The listing builds one solid part. Answer for the finished solid, in the listing's coordinates (mm). A direction names the side the tool comes from. Give positions to 0.01 mm unless a question says otherwise; leave off trailing zeros. Order: outer loops, then holes, each group sorted by start corner. A loop starts at its lowest first (then second) coordinate and runs counter-clockwise, first axis right, second up. Notation, with made-up numbers: (-33.5, -19) - (-14.5, -19) arc R26 cw to (-14.5, 3) - close; hole circle Ø7 at (79.5, 59). An arc over 180 degrees is marked (long way). Answer as CSV lines item,"result". Start each with the question number.
1. Flat-ended cylindrical pins translate along their axes: pin 1 (2.5 mm diameter, centred on y = 29.5, z = -2, fed in from +X); pin 2 (2 mm diameter, centred on y = 24, z = -3.5, fed in from +X); pin 3 (4 mm diameter, centred on x = -52, y = 2, fed in from +Z); pin 4 (7.5 mm diameter, centred on x = 64.79, y = 11.18, fed in from +Z). Find the tip coordinate at first contact, or state that the pin passes through.
2. Section A-A on x = -2.5 is taken. Give the vertices of the cut face in (y, z), and give its area (3 significant figures).
3. Determine the mould class of faces 6 (the flat face through (-11, 26.183, 17)), 7 (the cylindrical face through (63.872, 7.034, 1.479)), 8 (the cylindrical face through (79.79, 11.51, 1.48)), 9 (the flat face through (-60.207, 24, -2)) for opening direction Y: +Y half, -Y half, draft (parallel to the pull), parting line (faces both ways), or undercut.
4. Consider line 1 along Y through (x, z) = (-40, -8); line 2 along X through (y, z) = (23, -2.5); line 3 along X through (y, z) = (29, -10). Determine where each line is inside the solid, lowest interval first. Write a range as [from, to].
5. Section B-B on x = 66.5 is taken. Give the vertices of the cut face in (y, z).
6. Section D-D on y = 24 is taken. Give the vertices of the cut face in (x, z), and give its area (3 significant figures).
7. Which of the six approach directions +Z, -Z, +X, -X, +Y, -Y give full straight-line access (tool end or side, diameter ignored) to faces 1 (the flat face through (39.793, 24, 5)), 2 (the cylindrical face through (-100.203, 10.854, 1.479)), 3 (the flat face through (39.793, 24, -2)), 4 (the cylindrical face through (-86.128, 7.034, 1.479)), 5 (the flat face through (-60.207, 24, 5))?
8. Section C-C on z = -15 is taken. Give the vertices of the cut face in (x, y).
from build123d import *

# Parameters (mm, degrees)
ESBO_O1_R                = 4.25
RESSALTO_EXTRUS_O1_DEPTH = 3
ESBO_O2_W                = 150
ESBO_O2_H                = 50
RESSALTO_EXTRUS_O2_DEPTH = 5
RESSALTO_EXTRUS_O3_START = -25
RESSALTO_EXTRUS_O3_DEPTH = 100


with BuildPart() as part:
    # Esboço1 → Ressalto-extrusão1 (new body)
    with BuildSketch(Plane.XY):
        with BuildLine():
            Line((-85.207100592, 26.183431953), (64.792899408, 26.183431953))
            ThreePointArc((64.792899408, 26.183431953), (79.792899408, 11.183431953), (64.792899408, -3.816568047))
            Line((64.792899408, -3.816568047), (-85.207100592, -3.816568047))
            ThreePointArc((-85.207100592, -3.816568047), (-100.207100592, 11.183431953), (-85.207100592, 26.183431953))
        make_face()
        with Locations((-85.207100592, 11.183431953)):
            Circle(ESBO_O1_R, mode=Mode.SUBTRACT)
        with Locations((64.792899408, 11.183431953)):
            Circle(ESBO_O1_R, mode=Mode.SUBTRACT)
    extrude(amount=RESSALTO_EXTRUS_O1_DEPTH)

    # Esboço2 → Ressalto-extrusão2 (add)
    with BuildSketch(Plane(origin=(0, 26.183431953, 0), x_dir=(1, 0, 0), z_dir=(0, 1, 0))):
        with Locations((-10.207100592, -1.5)):
            Rectangle(ESBO_O2_W, ESBO_O2_H)
    extrude(amount=RESSALTO_EXTRUS_O2_DEPTH)

    # Esboço3 → Ressalto-extrusão3 (add)
    with BuildSketch(Plane.ZY.offset(85.207100592).offset(RESSALTO_EXTRUS_O3_START)):
        Polygon((3, 19.683431953), (9.5, 26.183431953), (3, 26.183431953), align=None)
        Polygon((0, 26.183431953), (0, 19.683431953), (-6.5, 26.183431953), align=None)
    extrude(amount=-RESSALTO_EXTRUS_O3_DEPTH)


solid = part.part
Checks:
1,pin 1,"stops at x = 64.79"
1,pin 2,"stops at x = 39.79"
1,pin 3,"stops at z = 3"
1,pin 4,"passes through"
2,outline,"(-3.82, 0) - (19.68, 0) - (26.18, -6.5) - (26.18, -23.5) - (31.18, -23.5) - (31.18, 26.5) - (26.18, 26.5) - (26.18, 9.5) - (19.68, 3) - (-3.82, 3) - close"
2,area,"382 mm²"
3,face 6,"-Y half"
3,face 7,"undercut"
3,face 8,"parting line"
3,face 9,"draft"
4,line 1,"y = [26.18, 31.18]"
4,line 2,"x = [-60.21, 39.79]"
4,line 3,"x = [-85.21, 64.79]"
5,outline,"(-3.72, 0) - (7.29, 0) - (7.29, 3) - (-3.72, 3) - close; (15.08, 0) - (26.09, 0) - (26.09, 3) - (15.08, 3) - close"
6,outline,"(-93, 0) - (-60.21, 0) - (-60.21, -4.32) - (39.79, -4.32) - (39.79, 0) - (72.59, 0) - (72.59, 3) - (39.79, 3) - (39.79, 7.32) - (-60.21, 7.32) - (-60.21, 3) - (-93, 3) - close"
6,area,"1,360 mm²"
7,face 1,"+Z, +X, -Y"
7,face 2,"+Z, -Z, -X"
7,face 3,"-Z, +X, -Y"
7,face 4,"+Z, -Z"
7,face 5,"+Z, -X, -Y"
8,outline,"(-85.21, 26.18) - (64.79, 26.18) - (64.79, 31.18) - (-85.21, 31.18) - close"
